Geometry: final body of the model. Coordinates: model frame, mm. A direction names the side the tool comes from. Round coordinates to 2 decimals unless told otherwise and drop trailing zeros.
from build123d import *

# Parameters (mm, degrees)
F0_W     = 89.5
F0_H     = 63
F1_DEPTH = 17
F2_DEPTH = 1
F3_R     = 1.5
F4_R     = 0.49999
F5_W     = 7.7
F5_H     = 5
F5_W_2   = 15.5
F5_H_2   = 5.6
F5_R     = 3.5
F6_DEPTH = 25
F7_W     = 59
F7_H     = 13.5
F7_H_2   = 3.5
F8_DEPTH = 25


# Not quite as in the source:
# - a fillet or chamfer is up to 0.001 mm smaller than in the source, because OpenCascade refuses the exact size


with BuildPart() as f1:
    # F0 (on Top) → F1 (new body)
    with BuildSketch(Plane.XY):
        Rectangle(F0_W, F0_H)
        Polygon((-42.75, 24.5), (-42.75, 29.5), (-37.75, 29.5), (37.75, 29.5), (42.75, 29.5), (42.75, 24.5), (42.75, -24.5), (42.75, -29.5), (37.75, -29.5), (-37.75, -29.5), (-42.75, -29.5), (-42.75, -24.5), align=None, mode=Mode.SUBTRACT)
    extrude(amount=F1_DEPTH)

    # F0 (on Top) → F2 (join)
    with BuildSketch(Plane.XY):
        Polygon((-0.0146734692, 1.6726181109), (-38.9898385852, 28.2601614148), (-40.9670818505, 26.2829181495), (-2.4649122807, 0), (-40.9670818505, -26.2829181495), (-38.9670818505, -28.2829181495), (0, -1.6826347305), (38.9670818505, -28.2829181495), (40.96658534, -26.28341466), (2.4510848657, -0.0094390737), (40.9670818505, 26.2829181495), (38.9670818505, 28.2829181495), align=None)
        Polygon((-37.75, 29.5), (-42.75, 29.5), (-42.75, 24.5), (-40.9670818505, 26.2829181495), (-38.9898385852, 28.2601614148), align=None)
        Polygon((42.75, 29.5), (37.75, 29.5), (38.9670818505, 28.2829181495), (40.9670818505, 26.2829181495), (42.75, 24.5), align=None)
        Polygon((42.75, -29.5), (42.75, -24.5), (40.96658534, -26.28341466), (38.9670818505, -28.2829181495), (37.75, -29.5), align=None)
        Polygon((-40.9670818505, -26.2829181495), (-42.75, -24.5), (-42.75, -29.5), (-37.75, -29.5), (-38.9670818505, -28.2829181495), align=None)
    extrude(amount=F2_DEPTH)

    # F3
    f3_edges = [f1.edges().sort_by_distance(p)[0] for p in [
        (0, 31.5, 17),
        (-44.75, 0, 17),
        (0, -31.5, 17),
        (44.75, 0, 17),
    ]]
    fillet(f3_edges, radius=F3_R)

    # F4 (radius 0.5 in the source; OpenCascade refuses exactly that, so slightly less here)
    f4_edges = [f1.edges().sort_by_distance(p)[0] for p in [
        (-19.502256, 14.96639, 1),
        (-21.715997, 13.141459, 1),
        (19.476204, 14.977768, 1),
        (21.709083, 13.13674, 1),
        (-21.715997, -13.141459, 1),
        (-19.483541, -14.982776, 0),
        (19.483541, -14.982776, 1),
        (21.708835, -13.146427, 1),
        (-41.858541, 25.391459, 1),
        (-38.369919, 28.880081, 1),
        (41.858541, 25.391459, 1),
        (38.358541, 28.891459, 1),
        (-41.858541, -25.391459, 1),
        (-38.358541, -28.891459, 1),
        (41.858293, -25.391707, 1),
        (38.358541, -28.891459, 1),
    ]]
    fillet(f4_edges, radius=F4_R)

    # F5 (on face) → F6 (cut)
    with BuildSketch(Plane(origin=(0, 31.5, 0), x_dir=(-1, 0, 0), z_dir=(0, 1, 0))):
        with Locations((-34.6, 5.8)):
            Rectangle(F5_W, F5_H)
        with Locations((-11, 7.8)):
            Rectangle(F5_W_2, F5_H_2)
        with Locations((11.0494399613, 7.5)):
            Circle(F5_R)
    extrude(amount=-F6_DEPTH, mode=Mode.SUBTRACT)

    # F7 (on face) → F8 (cut)
    with BuildSketch(Plane(origin=(-44.75, 0, 0), x_dir=(0, -1, 0), z_dir=(-1, 0, 0))):
        with Locations((0, 8.75)):
            Rectangle(F7_W, F7_H)
        with Locations((0, 17.25)):
            Rectangle(F7_W, F7_H_2)
    extrude(amount=-F8_DEPTH, mode=Mode.SUBTRACT)


solid = f1.part
1) Reachability of faces 1 (the flat face through (-1, -31.5, 8)), 2 (the flat face through (30.75, 31, 6)), 3 (the flat face through (44.75, 0, 8)), 4 (the flat face through (18.986, -14.643, 0.247)), 5 (the cylindrical face through (-19.974, 15.106, 0.857)) from +Z, -Z, +X, -X, +Y, -Y: full face, straight path, thin tool, end or side. Return the list, or none.
2) Draft query along Z for faces 6 (the flat face through (3.25, 31, 8)), 7 (the flat face through (-42.75, 0, 1)), 8 (the flat face through (11, 31, 5)), 9 (the cylindrical face through (-41.804, 25.659, 0.857)). Return one class per face: pulls with the +Z half, pulls with the -Z half, needs draft (parallel to the pull), parting line crosses it, or undercut.
3) Section A-A on x = 34. State how many separate pieces and enclosed holes the cut face has, plus the area to 3 significant figures.
4) Line query: probe 1 along Y at (x, z) = (22.5, 10.75); probe 2 along X at (y, z) = (-12, 1.75); probe 3 along Y at (x, z) = (14.5, 7.75). Output: solid intervals per line, ascending.
5) First-contact query: P1, Ø0.6, axis at x = 14.5, y = 30.5, coming from the -Z side; P2, Ø8.5, axis at y = 14, z = 10, coming from the -X side; P3, Ø1, axis at x = -43.5, y = -5.5, coming from the +Z side; P4, Ø10, axis at x = -35, y = -2, coming from the -Z side. Flat tips, straight axial feed; report the tip coordinate or a pass-through.
Filled in:
1. face 1: +Z, -Z, +X, -X, -Y
1. face 2: +Y
1. face 3: +Z, -Z, +X, +Y, -Y
1. face 4: +Z, -Z
1. face 5: +Z
2. face 6: undercut
2. face 7: needs draft
2. face 8: undercut
2. face 9: pulls with the +Z half
3. separate pieces: 5
3. enclosed holes: 0
3. area: 63.5 mm2
4. probe 1: y = -31.5 to -29.5, 29.5 to 31.5
4. probe 2: x = -44.75 to -42.75, 42.75 to 44.75
4. probe 3: y = -31.5 to -29.5
5. P1: stops at z = 0
5. P2: stops at x = 42.75
5. P3: stops at z = 2
5. P4: passes through
